Here's how the part is built. I have some questions about the finished solid (model axes, mm). A direction names the side the tool comes from. Round coordinates to 2 decimals unless told otherwise and drop trailing zeros. Loops run counter-clockwise (first coordinate to the right, second up) from the corner with the lowest first, then second, coordinate; pieces in that order, holes last. Notation, with made-up numbers: (-34, 56.25) - (-16, 56.25) arc R32 cw to (-16, 82.25) - close; hole circle Ø6 at (13.5, 20). An arc over 180 degrees is marked (long way). Answer as a JSON object with one key per item and string values. Group by question number.
1) I want a section at A-A, the plane z = 10. Please give me the cut outline in (x, y), then the cut area to 3 significant figures.
2) If I drill on line 1 along X through (y, z) = (-8, 13); line 2 along Z through (x, y) = (-9.5, -7.5), over which ranges is the centre line in solid material (lowest first)? Write a range as [from, to].
3) I want a section at B-B, the plane y = -11. Please give me the cut outline in (x, z), then the cut area to 3 significant figures.
4) Will these pins go through, and if not, where does the flat tip stop? P1, Ø1, axis at x = -12, y = 6, coming from the +Z side; P2, Ø6, axis at x = -14.5, z = 9, coming from the -Y side.
5) If we mould it in two halves opening along Y, with no side actions, what happens to faces 3 (the face through (18, 0, 9)), 4 (the face through (-16, -17, 9)), 5 (the face through (-18, 17, 9)), 6 (the face through (-0.1, 18.4, 17))? For each: pulls with the +Y half, pulls with the -Y half, needs draft (parallel to the pull), parting line crosses it, or undercut.
6) Which directions (+Z, -Z, +X, -X, +Y, -Y) give clear straight access to the entire face, cutting with the end or side of a thin tool? Please do faces 1 (the face through (0, 0, 0)), 2 (the face through (17, 16, 9)).
from build123d import *

# Parameters (mm, degrees)
F0_W     = 36
F0_H     = 36
F1_DEPTH = 1
F0_W_2   = 38
F0_H_2   = 38
F2_DEPTH = 17
F3_R     = 5


with BuildPart() as f1:
    # F0 (on Top) → F1 (new body)
    with BuildSketch(Plane.XY):
        Rectangle(F0_W, F0_H)
    extrude(amount=F1_DEPTH)

    # F0 (on Top) → F2 (join)
    with BuildSketch(Plane.XY):
        Rectangle(F0_W_2, F0_H_2)
        Rectangle(F0_W, F0_H, mode=Mode.SUBTRACT)
    extrude(amount=F2_DEPTH)

    # F3
    f3_edges = [f1.edges().sort_by_distance(p)[0] for p in [
        (-18, 18, 9),
        (18, 18, 9),
        (18, -18, 9),
        (-18, -18, 9),
        (-19, 19, 8.5),
        (-19, -19, 8.5),
        (19, -19, 8.5),
        (19, 19, 8.5),
    ]]
    fillet(f3_edges, radius=F3_R)


solid = f1.part
Outcome:
{
 "1": {"outline": "(-19, -14) arc R5 ccw to (-14, -19) - (14, -19) arc R5 ccw to (19, -14) - (19, 14) arc R5 ccw to (14, 19) - (-14, 19) arc R5 ccw to (-19, 14) - close; hole (-18, -13) arc R5 ccw to (-13, -18) - (13, -18) arc R5 ccw to (18, -13) - (18, 13) arc R5 ccw to (13, 18) - (-13, 18) arc R5 ccw to (-18, 13) - close", "area": "148 mm^2"},
 "2": {"line 1": "[-19, -18], [18, 19]", "line 2": "[0, 1]"},
 "3": {"outline": "(-19, 0) - (19, 0) - (19, 17) - (18, 17) - (18, 1) - (-18, 1) - (-18, 17) - (-19, 17) - close", "area": "70.0 mm^2"},
 "4": {"P1": "z = 1", "P2": "y = -19"},
 "5": {"face 3": "undercut", "face 4": "undercut", "face 5": "pulls with the +Y half", "face 6": "needs draft"},
 "6": {"face 1": "-Z, +X, -X, +Y, -Y", "face 2": "+Z"}
}
